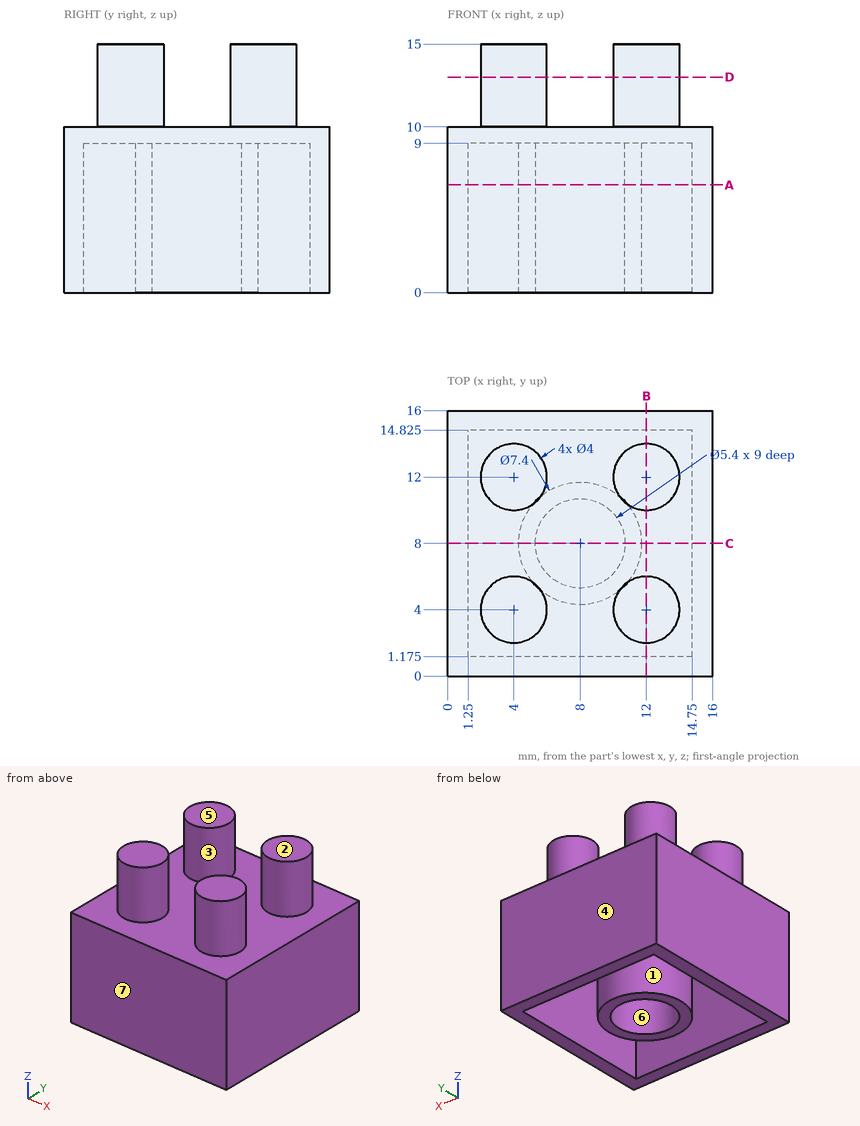
Verification items for this drawing (mm, ordinates from the low corner). A direction names the side the tool comes from. Coordinates: 2 decimals unless noted, no trailing zeros. Order: outer loops, then holes, each group sorted by start corner. A loop starts at its lowest first (then second) coordinate and runs counter-clockwise, first axis right, second up. Notation, with made-up numbers: (75.5, 7) - (81.5, 7) arc R23 ccw to (81.5, 16) - close; hole circle Ø1 at (-22, 12.5). An arc over 180 degrees is marked (long way). Answer in a Markdown table with one row per item. Add a question column.
1. Section check A-A (z = 6.5). Enter the section's corners in (x, y) (3 decimals).
2. Gauge pin test, flat ends, axial feed: pin 1 Ø1.5 at (x, z) = (9.5, 13) entering from +Y; pin 2 Ø2.5 at (x, y) = (8, 7) entering from -Z; pin 3 Ø1.5 at (y, z) = (10, 13) entering from +X. Record the tip position at first contact, or that the pin passes through.
3. Section check C-C (y = 8). Enter the section's corners in (x, z), plus the area to 3 significant figures.
4. Section check B-B (x = 12). Enter the section's corners in (y, z) (3 decimals).
5. Draft check along Y on the marked faces 4, 5, 6 and 7. Enter one of: +Y half, -Y half, draft (parallel to the pull), parting line (faces both ways), or undercut.
6. Material ranges on L1, parallel to Y at x = 8, z = 4 (3 decimals); L2, parallel to X at y = 4.25, z = 6.75; L3, parallel to Y at x = 5, z = 6 (1 decimal), recorded low to high. Write a range as [from, to].
7. Section check D-D (z = 13). Enter the section's corners in (x, y).
8. Access from +Z, -Z, +X, -X, +Y, -Y to the whole of each face (thin tool, end or side, straight path). Record for the marked faces 1, 2 and 3.
Data:
| question | item | result |
|---|---|---|
| 1 | outline | (0, 0) - (16, 0) - (16, 16) - (0, 16) - close; circle Ø7.4 at (8, 8); hole (1.25, 1.175) - (14.75, 1.175) - (14.75, 14.825) - (1.25, 14.825) - close; hole circle Ø5.4 at (8, 8) |
| 2 | pin 1 | stops at y = 12.97 |
| 2 | pin 2 | stops at z = 9 |
| 2 | pin 3 | stops at x = 13.56 |
| 3 | outline | (0, 0) - (1.25, 0) - (1.25, 9) - (4.3, 9) - (4.3, 0) - (5.3, 0) - (5.3, 9) - (10.7, 9) - (10.7, 0) - (11.7, 0) - (11.7, 9) - (14.75, 9) - (14.75, 0) - (16, 0) - (16, 10) - (0, 10) - close |
| 3 | area | 56.5 mm² |
| 4 | outline | (0, 0) - (1.175, 0) - (1.175, 9) - (14.825, 9) - (14.825, 0) - (16, 0) - (16, 10) - (14, 10) - (14, 15) - (10, 15) - (10, 10) - (6, 10) - (6, 15) - (2, 15) - (2, 10) - (0, 10) - close |
| 5 | face 4 | +Y half |
| 5 | face 5 | draft |
| 5 | face 6 | undercut |
| 5 | face 7 | -Y half |
| 6 | L1 | y = [0, 1.175], [4.3, 5.3], [10.7, 11.7], [14.825, 16] |
| 6 | L2 | x = [0, 1.25], [14.75, 16] |
| 6 | L3 | y = [0, 1.2], [5.8, 10.2], [14.8, 16] |
| 7 | outline | circle Ø4 at (4, 4); circle Ø4 at (4, 12); circle Ø4 at (12, 4); circle Ø4 at (12, 12) |
| 8 | face 1 | -Z |
| 8 | face 2 | +Z, +X, -X, +Y, -Y |
| 8 | face 3 | +Z |
